Part model, mm, in its own coordinate system. A direction names the side the tool comes from. Give positions to 0.01 mm unless a question says otherwise; leave off trailing zeros. Order: outer loops, then holes, each group sorted by start corner. A loop starts at its lowest first (then second) coordinate and runs counter-clockwise, first axis right, second up. Notation, with made-up numbers: M -28,-30.75 L -20,-30.75 A26 ccw -20,-0.75 Z; hole C 3.25,20 d4. An arc over 180 degrees is marked long. Write each question's results on one line, items separated by ' | '. Start each with the question number.
from build123d import *

# Parameters (mm, degrees)
F1_DEPTH = 25.4


with BuildPart() as f1:
    # F0 (on Top) → F1 (new body)
    with BuildSketch(Plane.XY):
        with BuildLine():
            Line((0, -19.6916791789), (0, 0))
            Line((0, 0), (19.6916791789, 0))
            ThreePointArc((19.6916791789, 0), (-13.9241198804, 13.9241198804), (0, -19.6916791789))
        make_face()
        with BuildLine():
            Line((19.6916791789, 0), (0, 0))
            Line((0, 0), (0, -19.6916791789))
            ThreePointArc((0, -19.6916791789), (13.9241198804, -13.9241198804), (19.6916791789, 0))
        make_face()
        with BuildLine():
            Line((53.0525743961, 0), (19.6916791789, 0))
            ThreePointArc((19.6916791789, 0), (13.9241198804, -13.9241198804), (0, -19.6916791789))
            Line((0, -19.6916791789), (0, -47.5333593786))
            Line((0, -47.5333593786), (53.0525743961, -47.5333593786))
            Line((53.0525743961, -47.5333593786), (53.0525743961, 0))
        make_face()
    extrude(amount=F1_DEPTH)


solid = f1.part
(1) Saw through at A-A on z = 12.75. Give the cut face in (x, y).
(2) Saw through at B-B on x = 25. Give the cut face in (y, z).
(3) Drop flat-ended pins along their axis: P1, Ø6, axis at y = -30.5, z = 5, coming from the -X side; P2, Ø7.5, axis at x = 32.5, z = 17.5, coming from the +Y side; P3, Ø12, axis at x = 13.5, z = 14, coming from the +Y side. Give the stop position or say it passes through.
(4) Tool access for faces 1 (the flat face through (37, 0, 13)), 2 (the flat face through (26, -47.533, 13)), 3 (the flat face through (0, -33, 13)): list every direction of +Z, -Z, +X, -X, +Y, -Y with a clear straight run to the whole face (end or side of a thin tool).
(5) Saw through at C-C on y = -40. Give the cut face in (x, z), plus the area to 3 significant figures.
(6) Probe L1, parallel to Y at x = 50, z = 11.5; L2, parallel to X at y = -20.5, z = 7.25; L3, parallel to Y at x = 7, z = 23. List the from-to ranges inside material, lowest first.
Taken from the geometry:
1) outline: M 0,-47.53 L 53.05,-47.53 L 53.05,0 L 19.69,0 A19.69 ccw long 0,-19.69 Z
2) outline: M -47.53,0 L 0,0 L 0,25.4 L -47.53,25.4 Z
3) P1: stops at x = 0 | P2: stops at y = 0 | P3: stops at y = 18.21
4) face 1: +Z, -Z, +X, +Y | face 2: +Z, -Z, +X, -X, -Y | face 3: +Z, -Z, -X, -Y
5) outline: M 0,0 L 53.05,0 L 53.05,25.4 L 0,25.4 Z | area: 1,350 mm²
6) L1: y = -47.53 to 0 | L2: x = 0 to 53.05 | L3: y = -47.53 to 18.41
